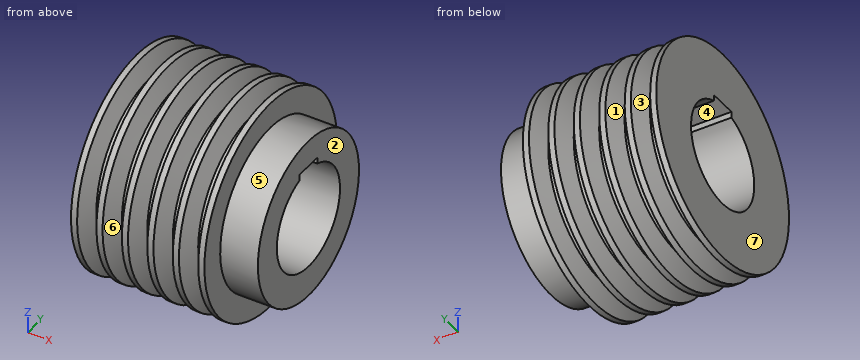
from build123d import *

# Parameters (mm, degrees)
F2_R     = 25
F3_DEPTH = 84
F5_DEPTH = 84


with BuildPart() as f1:
    # F0 (on Front) → F1 (revolve)
    with BuildSketch(Plane.XZ):
        Polygon((38.5438650846, 52.5), (38.5438650846, 0), (122.5438650846, 0), (122.5438650846, 40), (104.0438650846, 40), (104.0438650846, 52.5), (101.0438650846, 52.5), (97.7938650846, 42.5), (94.7938650846, 42.5), (91.5438650846, 52.5), (88.5438650846, 52.5), (85.2938650846, 42.5), (82.2938650846, 42.5), (79.0438650846, 52.5), (76.0438650846, 52.5), (72.7938650846, 42.5), (69.7938650846, 42.5), (66.5438650846, 52.5), (63.5438650846, 52.5), (60.2938650846, 42.5), (57.2938650846, 42.5), (54.0438650846, 52.5), (51.0438650846, 52.5), (47.7938650846, 42.5), (44.7938650846, 42.5), (41.5438650846, 52.5), align=None)
    revolve(axis=Axis((80.5438650846, 0, 0), (-1, 0, 0)))

    # F2 (on face) → F3 (cut)
    with BuildSketch(Plane.YZ.offset(122.5438650846)):
        Circle(F2_R)
    extrude(amount=-F3_DEPTH, mode=Mode.SUBTRACT)

    # F4 (on face) → F5 (cut)
    with BuildSketch(Plane.YZ.offset(122.5438650846)):
        with BuildLine():
            Line((-7, 27), (-7, 24))
            ThreePointArc((-7, 24), (0, 25), (7, 24))
            Line((7, 24), (7, 27))
            Line((7, 27), (-7, 27))
        make_face()
    extrude(amount=-F5_DEPTH, mode=Mode.SUBTRACT)


solid = f1.part
The listing builds one solid part. Answer for the finished solid, in the listing's coordinates (mm). Face numbers are marked on the shaded views. A direction names the side the tool comes from. Give positions to 0.01 mm unless a question says otherwise; leave off trailing zeros. Answer as a JSON object with one key per item and string values.
1. Flat-ended cylindrical pins translate along their axes: pin 1 Ø12 at (x, z) = (88, 28.5) entering from +Y; pin 2 Ø4 at (x, z) = (77, -27) entering from -Y; pin 3 Ø1 at (x, y) = (89.5, -22) entering from -Z. Find the tip coordinate at first contact, or state that the pin passes through.
Determined:
{"pin 1": "y = 47.42", "pin 2": "y = -46.17", "pin 3": "z = -47.9"}
2. Find the intervals of material crossed by L1, parallel to X at y = -19, z = 40; L2, parallel to X at y = -1, z = -44; L3, parallel to Y at x = 101.5, z = 0, in increasing order. Write a range as [from, to].
Determined:
{"L1": "[38.54, 44.21], [48.37, 56.71], [60.87, 69.21], [73.37, 81.71], [85.87, 94.21], [98.37, 104.04]", "L2": "[38.54, 44.3], [48.29, 56.8], [60.79, 69.3], [73.29, 81.8], [85.79, 94.3], [98.29, 104.04]", "L3": "[-52.5, -25], [25, 52.5]"}
3. A cutting plane is placed at A-A (z = 46). Give the number of separate pieces and of enclosed holes in the cut face, then the cut area to 3 significant figures.
Determined:
{"separate pieces": "6", "enclosed holes": "0", "area": "1,610 mm²"}
4. For a pull along X with two mould halves and no side action, classify the marked faces 1, 2, 3 and 4 as pulls with the +X half, pulls with the -X half, needs draft (parallel to the pull), parting line crosses it, or undercut.
Determined:
{"face 1": "undercut", "face 2": "pulls with the +X half", "face 3": "undercut", "face 4": "needs draft"}
5. For the marked faces 5, 6 and 7, determine the directions among +Z, -Z, +X, -X, +Y, -Y from which every point of the face is accessible in a straight line to the end or side of a thin tool.
Determined:
{"face 5": "+X", "face 6": "none", "face 7": "+Z, -Z, -X, +Y, -Y"}
